from build123d import *

# Parameters (mm, degrees)
SKETCH5_W           = 6.1595
SKETCH5_H           = 101.6
SKETCH5_W_2         = 101.6
SKETCH5_H_2         = 6.1595
BOSS_EXTRUDE1_DEPTH = 19.05


with BuildPart() as part:
    # Sketch2 → Loft1 section 0
    with BuildSketch(Plane(origin=(0, 127, 0), x_dir=(1, 0, 0), z_dir=(0, 1, 0))):
        with BuildLine():
            Line((-50.8, -50.8), (278.13, -50.8))
            Line((278.13, -50.8), (278.13, 276.352))
            Line((278.13, 276.352), (-50.8, 276.352))
            Line((-50.8, 276.352), (-50.8, -50.8))
        make_face()
    # Sketch1 → Loft1 section 1
    with BuildSketch(Plane(origin=(0, 0, 0), x_dir=(1, 0, 0), z_dir=(0, 1, 0))):
        with BuildLine():
            Line((0, 0), (227.33, 0))
            Line((227.33, 0), (227.33, 225.552))
            Line((227.33, 225.552), (0, 225.552))
            Line((0, 225.552), (0, 0))
        make_face()
    loft()

    # Sketch4 → Cut-Loft3 section 0
    with BuildSketch(Plane.XZ):
        with BuildLine():
            Line((208.28, -19.05), (19.05, -19.05))
            Line((19.05, -19.05), (19.05, -206.502))
            Line((19.05, -206.502), (208.28, -206.502))
            Line((208.28, -206.502), (208.28, -19.05))
        make_face()
    # Sketch3 → Cut-Loft3 section 1
    with BuildSketch(Plane(origin=(0, 127, 0), x_dir=(1, 0, 0), z_dir=(0, 1, 0))):
        with BuildLine():
            Line((-31.75, 257.302), (-31.75, -31.75))
            Line((-31.75, -31.75), (259.08, -31.75))
            Line((259.08, -31.75), (259.08, 257.302))
            Line((259.08, 257.302), (-31.75, 257.302))
        make_face()
    loft(mode=Mode.SUBTRACT)

    # Sketch5 → Boss-Extrude1 (add)
    with BuildSketch(Plane.XZ):
        with Locations((3.07975, -112.776)):
            Rectangle(SKETCH5_W, SKETCH5_H)
        with Locations((15.97025, -112.776)):
            Rectangle(SKETCH5_W, SKETCH5_H)
        with Locations((113.665, -3.07975)):
            Rectangle(SKETCH5_W_2, SKETCH5_H_2)
        with Locations((113.665, -15.97025)):
            Rectangle(SKETCH5_W_2, SKETCH5_H_2)
        with Locations((223.36125, -113.665)):
            Rectangle(SKETCH5_W, SKETCH5_H)
        with Locations((210.47075, -113.665)):
            Rectangle(SKETCH5_W, SKETCH5_H)
        with Locations((112.776, -223.36125)):
            Rectangle(SKETCH5_W_2, SKETCH5_H_2)
        with Locations((112.776, -210.47075)):
            Rectangle(SKETCH5_W_2, SKETCH5_H_2)
    extrude(amount=BOSS_EXTRUDE1_DEPTH)


solid = part.part
CAD build for the part. Positions are in the model's coordinates, mm. A direction names the side the tool comes from. Coordinates: 2 decimals unless noted, no trailing zeros. Use a Markdown table: item, result. Add a question column.
Item 1: Mould opens along X. For faces 5 (the face through (113, -9, 0)), 6 (the face through (207.391, -9, -114)), 7 (the face through (0, -9, -113)) say: pulls with the +X half, pulls with the -X half, needs draft (parallel to the pull), parting line crosses it, or undercut.
Item 2: Flat gauge pins, fed straight in: pin 1 (5 mm diameter, centred on y = -10, z = -16.5, fed in from +X) (3 decimals); pin 2 (8 mm diameter, centred on x = 102, y = 78.5, fed in from +Z); pin 3 (15 mm diameter, centred on y = -12, z = -102.5, fed in from -X). Where does each tip first touch, or does it go through?
Item 3: 3-axis set-ups, long thin cutter, end or side, ignore diameter. For faces 1 (the face through (226.441, -9, -114)), 2 (the face through (213.55, -9, -114)), 3 (the face through (113, -9, -6.16)), 4 (the face through (112, -9, -226.441)): which of +Z, -Z, +X, -X, +Y, -Y reach the whole face in a straight line?
Item 4: Drill centre lines: L1, parallel to Z at x = 151, y = -9.5; L2, parallel to Z at x = 62.5, y = -4; L3, parallel to X at y = 59.5, z = -29. Where is each one in solid material? Low to high. Write a range as from..to.
Numbers:
| question | item | result |
|---|---|---|
| 1 | face 5 | needs draft |
| 1 | face 6 | undercut |
| 1 | face 7 | pulls with the -X half |
| 2 | pin 1 | x = 164.465 |
| 2 | pin 2 | z = 33 |
| 2 | pin 3 | x = 0 |
| 3 | face 1 | +Z, -Z, +X, -Y |
| 3 | face 2 | +Z, -Z, -Y |
| 3 | face 3 | +X, -X, -Y |
| 3 | face 4 | -Z, +X, -X, -Y |
| 4 | L1 | -226.44..-220.28, -213.55..-207.39, -19.05..-12.89, -6.16..0 |
| 4 | L2 | -226.44..-220.28, -213.55..-207.39 |
| 4 | L3 | -23.8..-4.75, 232.08..251.13 |
